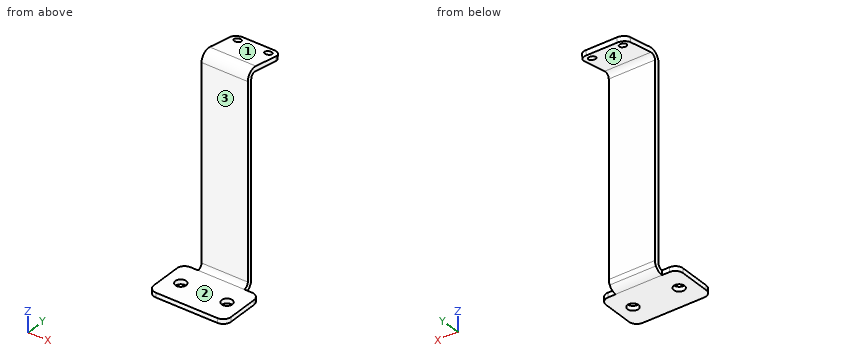
from build123d import *

# Parameters (mm, degrees)
SM_BASE_FLANGE_1_DEPTH = 3
HOLE_WIZARD_M61_D      = 7
OTHER_START            = -15
OTHER_1_DEPTH          = 30
OTHER_1_2_DEPTH        = 30
SM_EDGE_FLANGE_1_DEPTH = 30
HOLE_WIZARD_M41_D      = 4.5
HOLE_WIZARD_M41_DEPTH  = 3
FILLET_1_R             = 5
FILLET_2_R             = 5


# Read off the part's stored shape, not the designer's step: Нарисованный сгиб1
# Sheet-metal steps are written as plain solids
with BuildPart() as part:
    # Sketch 1 → Базовая кромка1 (new body)
    with BuildSketch(Plane.XY):
        Polygon((15, 30), (15, 162), (-15, 162), (-15, 30), (-25, 30), (-25, 0), (25, 0), (25, 30), align=None)
    extrude(amount=-SM_BASE_FLANGE_1_DEPTH)

    # Сверло под метчик  спиральное M61 (through all)
    with Locations(Plane.XY):
        with Locations((-15, 15), (15, 15)):
            Hole(HOLE_WIZARD_M61_D / 2)

    # Other 1 outline → Other 1 (cut)
    with BuildSketch(Plane.YZ.offset(OTHER_START)):
        with BuildLine():
            Line((162, 0), (35.196152423, 0))
            ThreePointArc((35.196152423, 0), (33, -2.196152423), (30, -3))
            Line((30, -3), (162, -3))
            Line((162, -3), (162, 0))
        make_face()
    extrude(amount=OTHER_1_DEPTH, mode=Mode.SUBTRACT)

    # Other 1 2 outline → Other 1 2 (add)
    with BuildSketch(Plane.YZ.offset(OTHER_START)):
        with BuildLine():
            Line((36, 3), (36, 127.931416529))
            Line((36, 127.931416529), (33, 127.931416529))
            Line((33, 127.931416529), (33, 3))
            ThreePointArc((33, 3), (32.121320344, 0.878679656), (30, 0))
            Line((30, 0), (35.196152423, 0))
            ThreePointArc((35.196152423, 0), (35.795554958, 1.447085729), (36, 3))
        make_face()
    extrude(amount=OTHER_1_2_DEPTH)

    # Ребро-кромка1 section (across the edge) → Ребро-кромка1 (add)
    with BuildSketch(Plane(origin=(-15, 36, 131.506677307), x_dir=(0, -0.17364817766692373, -0.9848077530122094), z_dir=(1, 0, 0))):
        with BuildLine():
            Line((-3, 3.575260778), (-3, 26.424739222))
            Line((-3, 26.424739222), (0, 26.424739222))
            Line((0, 26.424739222), (0, 3.575260778))
            ThreePointArc((0, 3.575260778), (1.071637171, 1.277127448), (3.520944533, 0.620837519))
            Line((3.520944533, 0.620837519), (4.041889066, -2.33358574))
            ThreePointArc((4.041889066, -2.33358574), (-0.856725658, -1.021005881), (-3, 3.575260778))
        make_face()
    extrude(amount=SM_EDGE_FLANGE_1_DEPTH)

    # Отверстие с зазором M41
    with Locations(Plane(origin=(0, 24.095443669, 136.652051617), x_dir=(1, 0, 0), z_dir=(0, 0.17364817766692325, 0.9848077530122094))):
        with Locations((-10, 34.041923465), (10, 34.041923465)):
            Hole(HOLE_WIZARD_M41_D / 2, depth=HOLE_WIZARD_M41_DEPTH)

    # Скругление1
    fillet_1_edges = [part.edges().sort_by_distance(p)[0] for p in [
        (-25, 0, -1.5),
        (25, 0, -1.5),
        (25, 30, -1.5),
        (-25, 30, -1.5),
    ]]
    fillet(fillet_1_edges, radius=FILLET_1_R)

    # Скругление2
    fillet_2_edges = [part.edges().sort_by_distance(p)[0] for p in [
        (-15, 62.283760324, 128.395281125),
        (15, 62.283760324, 128.395281125),
    ]]
    fillet(fillet_2_edges, radius=FILLET_2_R)


solid = part.part
CAD build for the part. Positions are in the model's coordinates, mm. Face numbers are marked on the shaded views. Give positions to 0.01 mm unless a question says otherwise; leave off trailing zeros. Write each loop counter-clockwise with the first axis right and the second up, starting at its lowest first coordinate (ties: lowest second). Pieces come first, ordered by that corner, then holes. Notation, with made-up numbers: (28, 55) -> (51, 55) arc R21 ccw to (51, 66) -> close; hole circle Ø5 at (-34, 41). An arc over 180 degrees is marked (long way). Return JSON: item names as keys, results as strings.
Item 1: Two-plate mould, pull along Y, no slides. Class the marked faces 1, 2, 3 and 4: +Y half, -Y half, draft (parallel to the pull), parting line (faces both ways), or undercut.
Answer below:
{"face 1": "+Y half", "face 2": "draft", "face 3": "-Y half", "face 4": "undercut"}
Item 2: Drill centre lines: probe 1 along Z at (x, y) = (-10, 4); probe 2 along Y at (x, z) = (-5, 24.5); probe 3 along Z at (x, y) = (-7.5, 37). Where is each one in solid material? Low to high.
Answer below:
{"probe 1": "z = -3 to 0", "probe 2": "y = 33 to 36", "probe 3": "z = 130.17 to 133.59"}
Item 3: Drop flat-ended pins along their axis: pin 1 (6 mm diameter, centred on y = 31, z = 117, fed in from +X); pin 2 (15 mm diameter, centred on x = 2, z = 48, fed in from -Y); pin 3 (9 mm diameter, centred on x = 15, y = 15, fed in from -Z); pin 4 (15 mm diameter, centred on x = -4.5, z = 51, fed in from +Y). Give the stop position or say it passes through.
Answer below:
{"pin 1": "stops at x = 15", "pin 2": "stops at y = 33", "pin 3": "stops at z = -3", "pin 4": "stops at y = 36"}
Item 4: Band-saw the part on C-C (z = 8.5). List the corners of the cut face in (x, y).
Answer below:
{"outline": "(-15, 33) -> (15, 33) -> (15, 36) -> (-15, 36) -> close"}
Item 5: Band-saw the part on A-A (y = 15). List the corners of the cut face in (x, z), then the cut area to 3 significant figures.
Answer below:
{"outline": "(-25, -3) -> (-18.5, -3) -> (-18.5, 0) -> (-25, 0) -> close; (-11.5, -3) -> (11.5, -3) -> (11.5, 0) -> (-11.5, 0) -> close; (18.5, -3) -> (25, -3) -> (25, 0) -> (18.5, 0) -> close", "area": "108 mm2"}
Item 6: Band-saw the part on D-D (y = 27). List the corners of the cut face in (x, z).
Answer below:
{"outline": "(-24.58, -3) -> (24.58, -3) -> (24.58, 0) -> (-24.58, 0) -> close"}
Item 7: Band-saw the part on B-B (x = 3). List the corners of the cut face in (y, z).
Answer below:
{"outline": "(0, -3) -> (30, -3) arc R6 ccw to (36, 3) -> (36, 127.93) arc R3 cw to (39.52, 130.89) -> (62.02, 126.92) -> (62.54, 129.87) -> (40.04, 133.84) arc R6 ccw to (33, 127.93) -> (33, 3) arc R3 cw to (30, 0) -> (0, 0) -> close"}
